Source: CAD feature listing. Evaluate the final solid. Frame: model axes, mm. A direction names the side the tool comes from. Give positions to 0.01 mm unless a question says otherwise; leave off trailing zeros. Write each loop counter-clockwise with the first axis right and the second up, starting at its lowest first coordinate (ties: lowest second). Pieces come first, ordered by that corner, then holes.
```python
from build123d import *

# Parameters (mm, degrees)
SKETCH1_R                = 2.667
BOSS_EXTRUDE1_DEPTH      = 2.54
BOSS_EXTRUDE7_DEPTH      = 9.779
BOSS_EXTRUDE7_DEPTH_BACK = 9.779
BOSS_EXTRUDE8_DEPTH      = 3.175
BOSS_EXTRUDE9_START      = -3.175
BOSS_EXTRUDE9_DEPTH      = 3.175
CUT_EXTRUDE1_DEPTH       = 66.415448629


with BuildPart() as part:
    # Sketch1 → Boss-Extrude1 (new body)
    with BuildSketch(Plane(origin=(0, 0, 0), x_dir=(1, 0, 0), z_dir=(0, 1, 0))):
        with BuildLine():
            Line((-9.779, -12.918471663), (9.779, -12.918471663))
            ThreePointArc((9.779, -12.918471663), (7.425363666, -6.824700874), (7.431379329, -0.292196741))
            Line((7.431379329, -0.292196741), (7.431379329, 16.796462376))
            ThreePointArc((7.431379329, 16.796462376), (0, 23.317357624), (-7.431379329, 16.796462376))
            Line((-7.431379329, 16.796462376), (-7.431379329, -0.57095897))
            ThreePointArc((-7.431379329, -0.57095897), (-7.47774388, -6.959075495), (-9.779, -12.918471663))
        make_face()
        with Locations(Location((0, 0, 0), (0, 0, 270))):
            Circle(SKETCH1_R, mode=Mode.SUBTRACT)
        with Locations(Location((0, 12.7, 0), (0, 0, 270))):
            Circle(SKETCH1_R, mode=Mode.SUBTRACT)
    extrude(amount=BOSS_EXTRUDE1_DEPTH)

    # Sketch2 → Boss-Extrude7 (add, two sides: drawn at the far end of the back side and taken through both)
    with BuildSketch(Plane(origin=(0, 0, 0), x_dir=(0, 0, -1), z_dir=(1, 0, 0)).offset(-BOSS_EXTRUDE7_DEPTH_BACK)):
        with BuildLine():
            Line((-60.416471663, 0), (-57.114471663, 0))
            ThreePointArc((-57.114471663, 0), (-37.556471663, 12.446), (-17.998471663, 0))
            Line((-17.998471663, 0), (-12.918471663, 0))
            Line((-12.918471663, 0), (-12.918471663, 2.54))
            Line((-12.918471663, 2.54), (-15.458471663, 2.54))
            ThreePointArc((-15.458471663, 2.54), (-38.750541785, 15.661341156), (-60.416471663, 0))
        make_face()
    extrude(amount=BOSS_EXTRUDE7_DEPTH + BOSS_EXTRUDE7_DEPTH_BACK)

    # Sketch8 → Boss-Extrude8 (add)
    with BuildSketch(Plane.ZY.offset(9.779)):
        with BuildLine():
            Line((21.095390289, 4.826), (54.017553037, 4.826))
            ThreePointArc((54.017553037, 4.826), (37.556471663, 12.446), (21.095390289, 4.826))
        make_face()
    extrude(amount=-BOSS_EXTRUDE8_DEPTH)

    # Sketch9 → Boss-Extrude9 (add)
    with BuildSketch(Plane(origin=(9.779, 0, 0), x_dir=(0, 0, -1), z_dir=(1, 0, 0)).offset(BOSS_EXTRUDE9_START)):
        with BuildLine():
            Line((-54.017553037, 4.826), (-21.095390289, 4.826))
            ThreePointArc((-21.095390289, 4.826), (-37.556471663, 12.446), (-54.017553037, 4.826))
        make_face()
    extrude(amount=BOSS_EXTRUDE9_DEPTH)

    # Sketch10 → Cut-Extrude1 (cut, through all)
    with BuildSketch(Plane.ZY.offset(9.779)):
        with BuildLine():
            Line((54.017553037, 4.826), (57.868824209, 4.826))
            ThreePointArc((57.868824209, 4.826), (59.275844237, 2.483314384), (60.416471663, 0))
            Line((60.416471663, 0), (57.114471663, 0))
            ThreePointArc((57.114471663, 0), (55.726945646, 2.516273378), (54.017553037, 4.826))
        make_face()
    extrude(amount=-CUT_EXTRUDE1_DEPTH, mode=Mode.SUBTRACT)


solid = part.part
```
1. Section query D-D (z = 40.5). Return loops of the section in (x, y).
2. Section query B-B (x = 0). Return loops of the section in (y, z), plus the area to 3 significant figures.
3. Access query for faces 1 (the flat face through (-7, 4.826, 43)), 2 (the flat face through (6.604, 8, 38)), 3 (the flat face through (7.431, 1, -8)), 4 (the flat face through (0, 2.54, -4)). Directions: +Z, -Z, +X, -X, +Y, -Y. A direction counts if a zero-diameter tool reaches every point of the face in a straight line with its end or side. Return the directions, or none.
4. Pin query (flat end, axial travel): P1, Ø3, axis at y = 1, z = -8, coming from the +X side; P2, Ø3, axis at x = 2, y = 5, coming from the -Z side; P3, Ø5, axis at x = -5, z = 42, coming from the +Y side. Return the tip coordinate at first contact, or that it passes through.
5. Pull-direction query (X, two-part tool) for faces 5 (the flat face through (-6.604, 8, 37)), 6 (the cylindrical face through (7.442, 1.252, 6.915)), 7 (the flat face through (-7.431, 1, -8)); classes: pulls with the +X half, pulls with the -X half, needs draft (parallel to the pull), parting line crosses it, or undercut.
6. Line query: probe 1 along X at (y, z) = (0.6, -12.7); probe 2 along X at (y, z) = (5, 36); probe 3 along Y at (x, z) = (7.5, 10.5). Output: solid intervals per line, ascending.
7. Section query C-C (y = 10.5). Return loops of the section in (x, z), plus the area to 3 significant figures.
8. Section query A-A (z = -12.7). Return loops of the section in (x, y).
The answers:
1. outline: (-9.78, 4.83) - (-6.6, 4.83) - (-6.6, 12.24) - (6.6, 12.24) - (6.6, 4.83) - (9.78, 4.83) - (9.78, 15.5) - (-9.78, 15.5) - close
2. outline: (0, -23.32) - (2.54, -23.32) - (2.54, -15.37) - (0, -15.37) - close; (0, -10.03) - (2.54, -10.03) - (2.54, -2.67) - (0, -2.67) - close; (0, 2.67) - (2.54, 2.67) - (2.54, 15.46) arc R24.79 ccw to (4.83, 57.87) - (4.83, 54.02) arc R21.59 cw to (0, 18) - close
2. area: 228 mm2
3. face 1: +Z, +X, -X, -Y
3. face 2: -Y
3. face 3: -Z, +X, +Y, -Y
3. face 4: -Z, +X, -X, +Y
4. P1: stops at x = 7.43
4. P2: stops at z = 16
4. P3: stops at y = 15.61
5. face 5: undercut
5. face 6: pulls with the +X half
5. face 7: pulls with the -X half
6. probe 1: x = -7.43 to -2.67, 2.67 to 7.43
6. probe 2: x = -9.78 to -6.6, 6.6 to 9.78
6. probe 3: y = 0 to 2.54
7. outline: (-9.78, 22.16) - (9.78, 22.16) - (9.78, 52.54) - (-9.78, 52.54) - close; hole (-6.6, 28.6) - (6.6, 28.6) - (6.6, 46.51) - (-6.6, 46.51) - close
7. area: 358 mm2
8. outline: (-7.43, 0) - (-2.67, 0) - (-2.67, 2.54) - (-7.43, 2.54) - close; (2.67, 0) - (7.43, 0) - (7.43, 2.54) - (2.67, 2.54) - close
